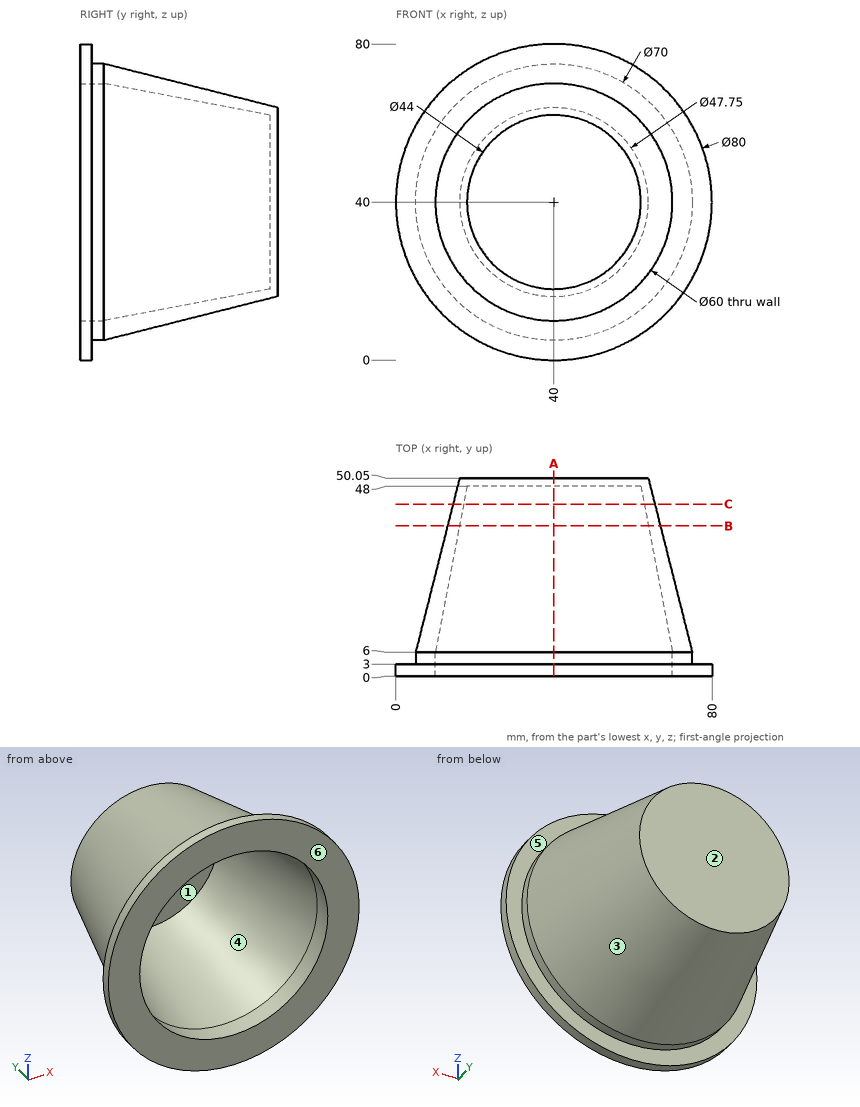
Here's the drawing with two shaded views (mm, measured from the low corner). I have some questions. A direction names the side the tool comes from. Round coordinates to 2 decimals unless told otherwise and drop trailing zeros. Order: outer loops, then holes, each group sorted by start corner. A loop starts at its lowest first (then second) coordinate and runs counter-clockwise, first axis right, second up. Notation, with made-up numbers: M -18.5,43 L 15.5,43 A23 cw 15.5,69 Z; hole C 47,74 d9. An arc over 180 degrees is marked long. Answer in a Markdown table with one row per item.
Item 1: If I drill on L1, parallel to Z at x = 40, y = 1; L2, parallel to Z at x = 40, y = 4.5; L3, parallel to X at y = 37, z = 24, over which ranges is the centre line in solid material (lowest first)? Write a range as from..to.
A:
| item | result |
|---|---|
| L1 | z = 0..10, 70..80 |
| L2 | z = 5..10, 70..75 |
| L3 | x = 18.04..21.98, 58.02..61.96 |
Item 2: Imagine slicing it at A-A, the plane x = 40. Write out the boundary of the cut face in (y, z) (3 decimals).
A:
| item | result |
|---|---|
| outline | M 0,0 L 3,0 L 3,5 L 6,5 L 50.05,16.125 L 50.05,63.875 L 6,75 L 3,75 L 3,80 L 0,80 L 0,70 L 6,70 L 48,62 L 48,18 L 6,10 L 0,10 Z |
Item 3: Imagine slicing it at C-C, the plane y = 43.5. Write out the boundary of the cut face in (x, z).
A:
| item | result |
|---|---|
| outline | C 40,40 d51.06; hole C 40,40 d45.71 |
Item 4: For the marked faces 5 and 6, which set-ups out of +Z, -Z, +X, -X, +Y, -Y let a thin tool reach every point of the face, with its end or its side?
A:
| item | result |
|---|---|
| face 5 | +Y |
| face 6 | +Z, -Z, +X, -X, -Y |
Item 5: Imagine slicing it at B-B, the plane y = 38. Write out the boundary of the cut face in (x, z).
A:
| item | result |
|---|---|
| outline | C 40,40 d53.84; hole C 40,40 d47.81 |
Item 6: I'm going to push flat-ended pins straight in: pin 1 (5 mm diameter, centred on x = 66, y = 26.5, fed in from -Z); pin 2 (1 mm diameter, centred on x = 44, y = 27.5, fed in from -Z); pin 3 (2 mm diameter, centred on x = 30, y = 30.5, fed in from -Z); pin 4 (3 mm diameter, centred on x = 59.5, z = 56, fed in from +Y). Where does each tip first touch, or does it pass through?
A:
| item | result |
|---|---|
| pin 1 | stops at z = 21.48 |
| pin 2 | stops at z = 10.56 |
| pin 3 | stops at z = 12.54 |
| pin 4 | stops at y = 50.05 |
Item 7: Thinking about a two-plate mould opening in X: for the marked faces 1, 2, 3 and 4, which applies, +X half, -X half, draft (parallel to the pull), parting line (faces both ways), or undercut?
A:
| item | result |
|---|---|
| face 1 | undercut |
| face 2 | draft |
| face 3 | parting line |
| face 4 | undercut |
